Source: CAD feature listing. Evaluate the final solid. Frame: model axes, mm. A direction names the side the tool comes from. Round coordinates to 2 decimals unless told otherwise and drop trailing zeros. Loops run counter-clockwise (first coordinate to the right, second up) from the corner with the lowest first, then second, coordinate; pieces in that order, holes last. Notation, with made-up numbers: (37.25, -35) - (71.25, -35) arc R25 ccw to (71.25, -21) - close; hole circle Ø3 at (14, 10.25). An arc over 180 degrees is marked (long way). One line per question, with ' | ' between items.
from build123d import *

# Parameters (mm, degrees)
SKETCH1_R               = 4.5
SKETCH1_R_2             = 4
SKETCH1_R_3             = 3.3
BOSS_EXTRUDE1_DEPTH     = 1.5
CUT_EXTRUDE1_DEPTH      = 7.538348415
CIRPATTERN1_COUNT       = 16
CUT_EXTRUDE2_DEPTH      = 7.478682276
CUT_EXTRUDE2_DEPTH_BACK = 7.478682276
SKETCH4_R               = 1.5
SKETCH5_R               = 3.05
SKETCH5_R_2             = 1.5
BOSS_EXTRUDE2_DEPTH     = 4


with BuildPart() as part:
    # Sketch1 → Boss-Extrude1 (new, symmetric)
    # profile 1 of 3: a face of its own
    with BuildSketch(Plane(origin=(0, 0, 0), x_dir=(1, 0, 0), z_dir=(0, 1, 0))):
        with Locations(Location((0, 0, 0), (0, 0, 270))):
            Circle(SKETCH1_R)
        Circle(SKETCH1_R_2, mode=Mode.SUBTRACT)
    # profile 2 of 3: a face of its own
    with BuildSketch(Plane(origin=(0, 0, 0), x_dir=(1, 0, 0), z_dir=(0, 1, 0))):
        Circle(SKETCH1_R_2)
        Circle(SKETCH1_R_3, mode=Mode.SUBTRACT)
    # profile 3 of 3: a face of its own
    with BuildSketch(Plane(origin=(0, 0, 0), x_dir=(1, 0, 0), z_dir=(0, 1, 0))):
        Circle(SKETCH1_R_3)
    extrude(amount=BOSS_EXTRUDE1_DEPTH, both=True)

    # Sketch3 → Cut-Extrude1 (cut, symmetric)
    with BuildSketch(Plane(origin=(0, 0, 0), x_dir=(1, 0, 0), z_dir=(0, 1, 0))):
        with BuildLine():
            ThreePointArc((-1.819764324, 5.475523519), (-0.723130395, 4.605944889), (-0.243947252, 3.290970942))
            ThreePointArc((-0.243947252, 3.290970942), (0, 3.3), (0.243947252, 3.290970942))
            ThreePointArc((0.243947252, 3.290970942), (0.723130395, 4.605944889), (1.819764324, 5.475523519))
            ThreePointArc((1.819764324, 5.475523519), (0, 5.77), (-1.819764324, 5.475523519))
        make_face()
    cut_extrude1 = extrude(amount=CUT_EXTRUDE1_DEPTH, both=True, mode=Mode.SUBTRACT)

    # CirPattern1: Cut-Extrude1 ×16 about axis
    cirpattern1_axis = Axis((0, 0, 0), (0, 1, 0))
    for i in range(1, CIRPATTERN1_COUNT):
        add(cut_extrude1.rotate(cirpattern1_axis, i * 360 / CIRPATTERN1_COUNT), mode=Mode.SUBTRACT)

    # Sketch4 → Cut-Extrude2 (cut, two sides: drawn at the far end of the back side and taken through both)
    with BuildSketch(Plane(origin=(0, 0, 0), x_dir=(1, 0, 0), z_dir=(0, 1, 0)).offset(-CUT_EXTRUDE2_DEPTH_BACK)):
        with Locations(Location((0, 0, 0), (0, 0, 270))):
            Circle(SKETCH4_R)
    extrude(amount=CUT_EXTRUDE2_DEPTH + CUT_EXTRUDE2_DEPTH_BACK, mode=Mode.SUBTRACT)

    # Sketch5 → Boss-Extrude2 (add)
    with BuildSketch(Plane(origin=(0, 1.5, 0), x_dir=(1, 0, 0), z_dir=(0, 1, 0))):
        with Locations(Location((0, 0, 0), (0, 0, 270))):
            Circle(SKETCH5_R)
        with Locations(Location((0, 0, 0), (0, 0, 270))):
            Circle(SKETCH5_R_2, mode=Mode.SUBTRACT)
    extrude(amount=BOSS_EXTRUDE2_DEPTH)


solid = part.part
1. Mould query, pull axis Z, two halves, no side actions, for faces 1 (the cylindrical face through (-0.36, 0.02, 3.89)), 2 (the cylindrical face through (-1.832, 0.021, -3.468)), 3 (the cylindrical face through (-3.468, 0.021, 1.832)). Classes: released by +Z, released by -Z, zero draft, split by the parting line, or undercut.
Worked out:
face 1: released by +Z | face 2: released by -Z | face 3: undercut
2. Section query A-A, the plane z = 0. Return loops of the section in (x, y).
Worked out:
outline: (-3.3, -1.5) - (-1.5, -1.5) - (-1.5, 5.5) - (-3.05, 5.5) - (-3.05, 1.5) - (-3.3, 1.5) - close; (1.5, -1.5) - (3.3, -1.5) - (3.3, 1.5) - (3.05, 1.5) - (3.05, 5.5) - (1.5, 5.5) - close
3. Section query D-D, the plane y = 4.25. Return loops of the section in (x, z).
Worked out:
outline: circle Ø6.1 at (0, 0); hole circle Ø3 at (0, 0)
4. Section query B-B, the plane x = 0. Return loops of the section in (y, z).
Worked out:
outline: (-1.5, -3.3) - (1.5, -3.3) - (1.5, -3.05) - (5.5, -3.05) - (5.5, -1.5) - (-1.5, -1.5) - close; (-1.5, 1.5) - (5.5, 1.5) - (5.5, 3.05) - (1.5, 3.05) - (1.5, 3.3) - (-1.5, 3.3) - close
5. Section query C-C, the plane x = 3.75. Return loops of the section in (y, z), plus the area to 4 significant figures.
Worked out:
outline: (-1.5, -2.49) - (1.5, -2.49) - (1.5, -2.12) - (-1.5, -2.12) - close; (-1.5, -1.16) - (1.5, -1.16) - (1.5, -0.32) - (-1.5, -0.32) - close; (-1.5, 0.32) - (1.5, 0.32) - (1.5, 1.16) - (-1.5, 1.16) - close; (-1.5, 2.12) - (1.5, 2.12) - (1.5, 2.49) - (-1.5, 2.49) - close | area: 7.245 mm2
6. Contact query for a flat-ended pin moving along its axis: P1, Ø3, axis at y = 4, z = 0, coming from the +X side. Output: stop coordinate, or through.
Worked out:
P1: stops at x = 3.05
7. Access query for faces 4 (the flat face through (-3, 1.5, -2)), 5 (the cylindrical face through (0.366, 0.021, 3.905)), 6 (the cylindrical face through (-2.503, 0.021, 3.02)), 7 (the cylindrical face through (-3.905, 0.021, 0.366)), 8 (the cylindrical face through (1.821, 0.021, -3.455)). Directions: +Z, -Z, +X, -X, +Y, -Y. A direction counts if a zero-diameter tool reaches every point of the face in a straight line with its end or side. Return the directions, or none.
Worked out:
face 4: +Y | face 5: +Z, +Y, -Y | face 6: +Y, -Y | face 7: -X, +Y, -Y | face 8: -Z, +Y, -Y
8. Material intervals for probe 1 along X at (y, z) = (2.25, 0); probe 2 along Z at (x, y) = (3.5, -0.75); probe 3 along Z at (x, y) = (0, 1), sorted ascending.
Worked out:
probe 1: x = -3.05 to -1.5, 1.5 to 3.05 | probe 2: z = -2.69 to -1.86, -1.13 to -0.27, 0.27 to 1.13, 1.86 to 2.69 | probe 3: z = -3.3 to -1.5, 1.5 to 3.3
